Check sheet for the drawn part. Datum: minimum x, y, z corner. Units: mm. A direction names the side the tool comes from. Coordinates: 2 decimals unless noted, no trailing zeros. Order: outer loops, then holes, each group sorted by start corner. A loop starts at its lowest first (then second) coordinate and runs counter-clockwise, first axis right, second up. Notation, with made-up numbers: (88.25, 69.25) - (128.25, 69.25) arc R14 ccw to (128.25, 90.25) - close; hole circle Ø2 at (-36.75, 60.5). An arc over 180 degrees is marked (long way). Put each result on its own line as item: value.
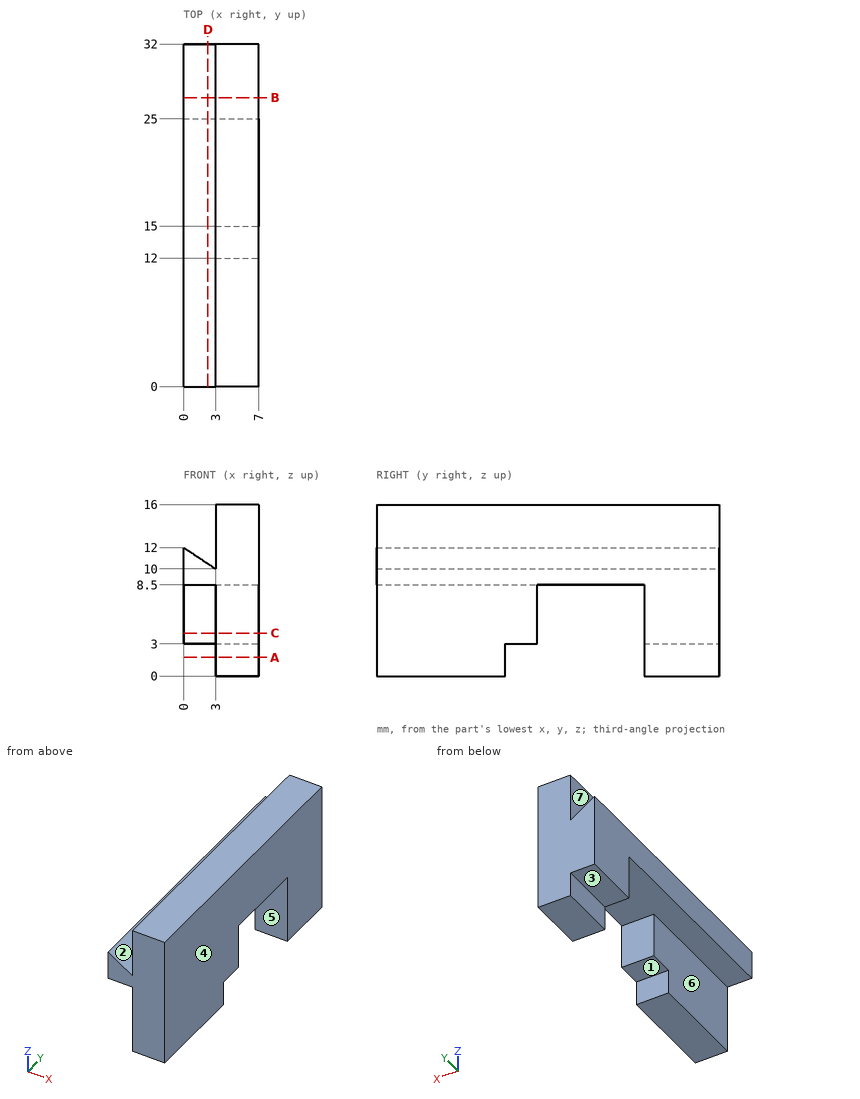
Q1. Draft check along X on the marked faces 5, 6 and 7. Enter one of: pulls with the +X half, pulls with the -X half, needs draft (parallel to the pull), parting line crosses it, or undercut.
Answer block:
face 5: needs draft
face 6: pulls with the -X half
face 7: undercut
Q2. Depth check by flat-ended pin: pin 1 Ø1.5 at (x, y) = (1.5, 28.5) entering from -Z; pin 2 Ø2.5 at (y, z) = (5.5, 6.5) entering from -X; pin 3 Ø3.5 at (x, y) = (4, 17) entering from -Z. Enter the tip coordinate at first touch or a pass-through.
Answer block:
pin 1: stops at z = 3
pin 2: stops at x = 3
pin 3: stops at z = 8.5
Q3. Section check D-D on x = 2.25. Record the boundary of the cut face in (y, z), then the cut area to 4 significant figures.
Answer block:
outline: (0, 8.5) - (25, 8.5) - (25, 3) - (32, 3) - (32, 10.5) - (0, 10.5) - close
area: 102.5 mm^2
Q4. Access from +Z, -Z, +X, -X, +Y, -Y to the whole of each face (thin tool, end or side, straight path). Record for the marked faces 1, 2, 3 and 4.
Answer block:
face 1: -Z, +X, -X
face 2: +Z, +Y, -Y
face 3: -Z, -X, +Y, -Y
face 4: +Z, -Z, +X, +Y, -Y
Q5. Section check C-C on z = 4. Record the boundary of the cut face in (x, y).
Answer block:
outline: (0, 25) - (7, 25) - (7, 32) - (0, 32) - close; (3, 0) - (7, 0) - (7, 15) - (3, 15) - close
Q6. Section check A-A on z = 1.75. Record the boundary of the cut face in (x, y).
Answer block:
outline: (3, 0) - (7, 0) - (7, 12) - (3, 12) - close; (3, 25) - (7, 25) - (7, 32) - (3, 32) - close
Q7. Section check B-B on y = 27. Record the boundary of the cut face in (x, z).
Answer block:
outline: (0, 3) - (3, 3) - (3, 0) - (7, 0) - (7, 16) - (3, 16) - (3, 10) - (0, 12) - close
Q8. Thickness scan on L1, parallel to Y at x = 5, z = 6.5; L2, parallel to X at y = 4, z = 7.75; L3, parallel to Y at x = 0.75, z = 3.25. Record the ranges inside material, lowest first. Write a range as [from, to].
Answer block:
L1: y = [0, 15], [25, 32]
L2: x = [3, 7]
L3: y = [25, 32]
